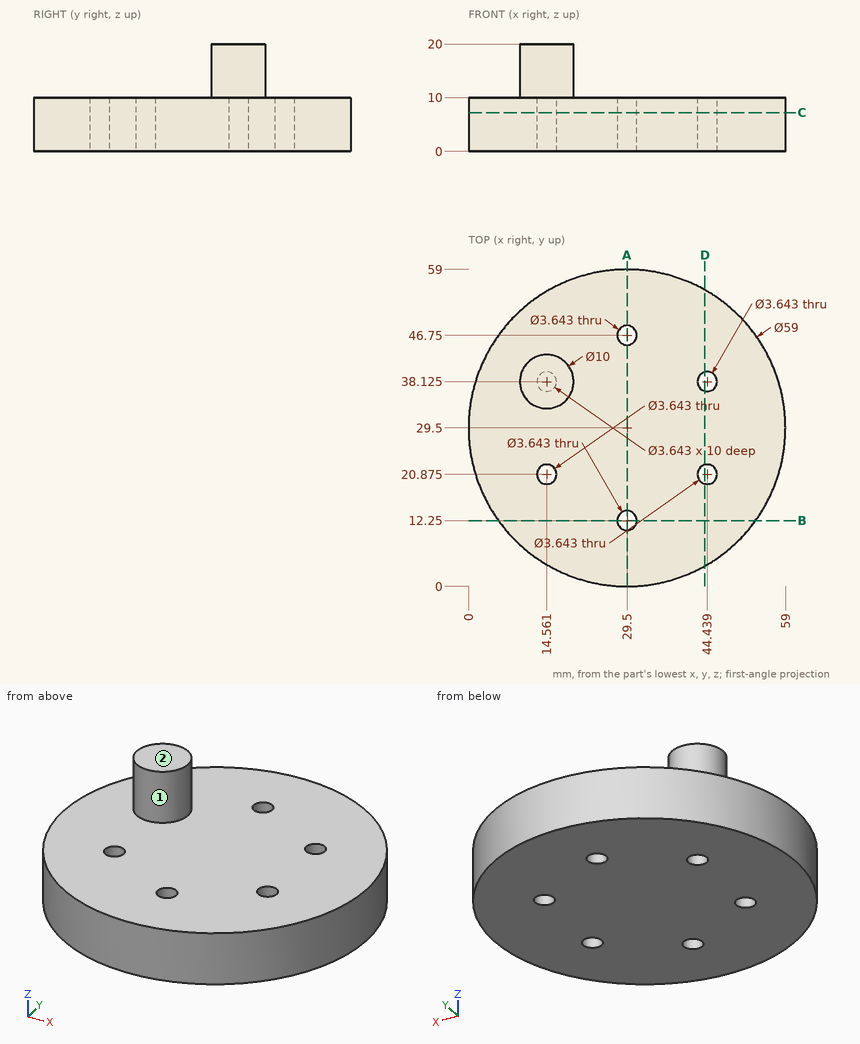
Geometry: see drawing. Coordinates: mm, zero at the bounding-box minimum. A direction names the side the tool comes from. Coordinates: 2 decimals unless noted, no trailing zeros. Loops run counter-clockwise (first coordinate to the right, second up) from the corner with the lowest first, then second, coordinate; pieces in that order, holes last. Notation, with made-up numbers: (-20.75, 86.5) - (-11.75, 86.5) arc R34 ccw to (-11.75, 121.5) - close; hole circle Ø2 at (7, -15). An arc over 180 degrees is marked (long way). Return JSON: item names as keys, results as strings.
Q1. Material intervals for line 1 along Y through (x, z) = (29.5, 2.5); line 2 along Y through (x, z) = (45.5, 7.5) (1 decimal); line 3 along Z through (x, y) = (18.5, 14.5), sorted ascending.
Results:
{"line 1": "0 to 10.43, 14.07 to 44.93, 48.57 to 59", "line 2": "4.7 to 19.4, 22.4 to 36.6, 39.6 to 54.3", "line 3": "0 to 10"}
Q2. Section A-A, the plane x = 29.5. Return loops of the section in (y, z).
Results:
{"outline": "(0, 0) - (10.43, 0) - (10.43, 10) - (0, 10) - close; (14.07, 0) - (44.93, 0) - (44.93, 10) - (14.07, 10) - close; (48.57, 0) - (59, 0) - (59, 10) - (48.57, 10) - close"}
Q3. Section C-C, the plane z = 7.25. Give the number of separate pieces and of enclosed holes in the cut face, plus the area to 3 significant figures.
Results:
{"separate pieces": "1", "enclosed holes": "6", "area": "2,670 mm2"}
Q4. Section B-B, the plane y = 12.25. Return loops of the section in (x, z), plus the area to 3 significant figures.
Results:
{"outline": "(5.57, 0) - (27.68, 0) - (27.68, 10) - (5.57, 10) - close; (31.32, 0) - (53.43, 0) - (53.43, 10) - (31.32, 10) - close", "area": "442 mm2"}
Q5. Section D-D, the plane x = 44. Return loops of the section in (y, z), plus the area to 3 significant figures.
Results:
{"outline": "(3.81, 0) - (19.11, 0) - (19.11, 10) - (3.81, 10) - close; (22.64, 0) - (36.36, 0) - (36.36, 10) - (22.64, 10) - close; (39.89, 0) - (55.19, 0) - (55.19, 10) - (39.89, 10) - close", "area": "443 mm2"}
Q6. Contact query for flat-ended pins moving along their axis: P1, Ø3, axis at x = 14.56, y = 20.88, coming from the -Z side; P2, Ø2, axis at x = 25.5, z = 8, coming from the -Y side; P3, Ø2, axis at x = 45.5, y = 27.5, coming from the +Z side; P4, Ø10, axis at x = 48, z = 2.5, coming from the -Y side. Output: stop coordinate, or through.
Results:
{"P1": "through", "P2": "y = 0.15", "P3": "z = 10", "P4": "y = 3.27"}
Q7. Access query for the marked faces 1 and 2. Directions: +Z, -Z, +X, -X, +Y, -Y. A direction counts if a zero-diameter tool reaches every point of the face in a straight line with its end or side. Return the directions, or none.
Results:
{"face 1": "+Z", "face 2": "+Z, +X, -X, +Y, -Y"}
